Drawing for the job (mm, zero at the part's lowest x, y, z). A direction names the side the tool comes from. Give positions to 0.01 mm unless a question says otherwise; leave off trailing zeros. Write each loop counter-clockwise with the first axis right and the second up, starting at its lowest first coordinate (ties: lowest second). Pieces come first, ordered by that corner, then holes. Notation, with made-up numbers: (85, -24) - (127, -24) arc R25 ccw to (127, -3) - close; hole circle Ø2 at (77.5, 83.5). An arc over 180 degrees is marked (long way). Write item = value, one per line. Start each with the question number.
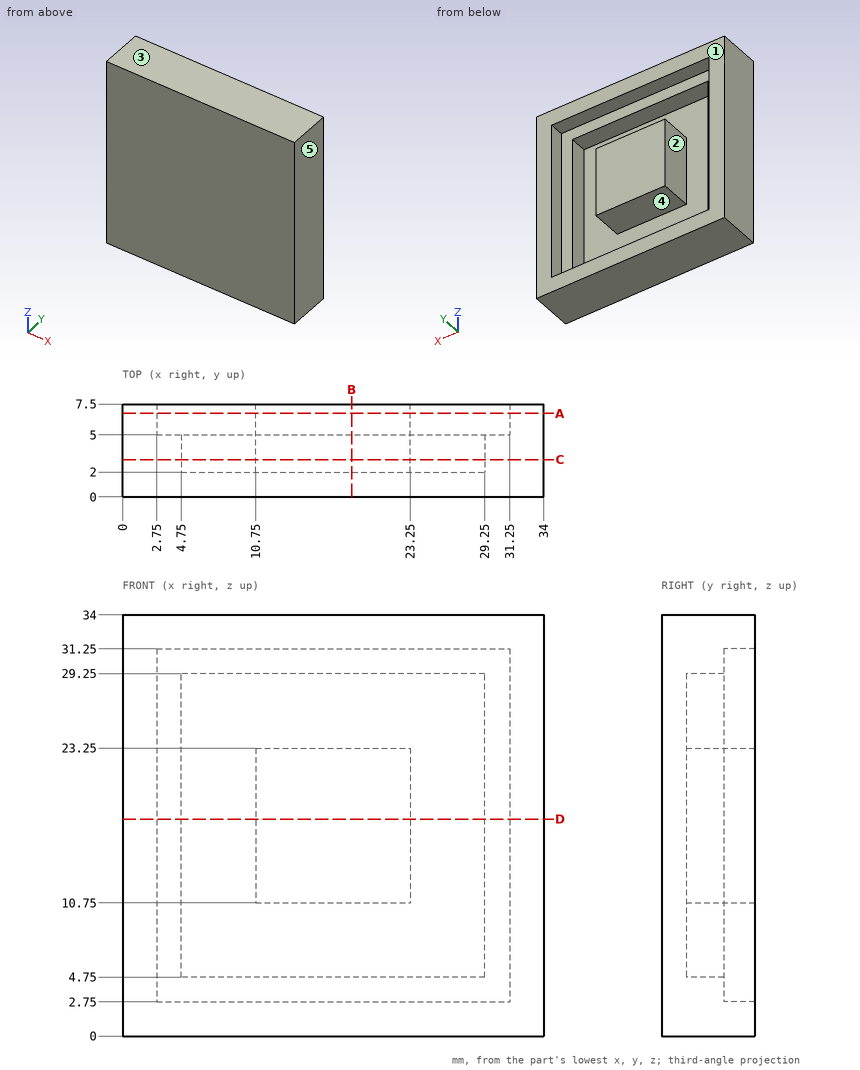
1. Cut at B-B (x = 18.5). Give the cut face in (y, z), then the cut area to 3 significant figures.
2. Tool access for the marked faces 1 and 2: list every direction of +Z, -Z, +X, -X, +Y, -Y with a clear straight run to the whole face (end or side of a thin tool).
3. Wall check: line 1 along X through (y, z) = (7.25, 14.5); line 2 along Z through (x, y) = (17, 4.5). Give the ranges that are in metal, low to high.
4. Cut at D-D (z = 17.5). Give the cut face in (x, y).
5. Pin check, flat tip, straight feed: pin 1 Ø3.5 at (x, y) = (17, 4) entering from -Z. Stop position of the tip, or through.
6. Cut at A-A (y = 6.75). Give the cut face in (x, z).
7. Cut at C-C (y = 3). Give the cut face in (x, z), then the cut area to 3 significant figures.
8. Mould opens along X. For the marked faces 3, 4 and 5 say: +X half, -X half, draft (parallel to the pull), parting line (faces both ways), or undercut.
Output:
q1.outline = (0, 0) - (7.5, 0) - (7.5, 2.75) - (5, 2.75) - (5, 4.75) - (2, 4.75) - (2, 10.75) - (7.5, 10.75) - (7.5, 23.25) - (2, 23.25) - (2, 29.25) - (5, 29.25) - (5, 31.25) - (7.5, 31.25) - (7.5, 34) - (0, 34) - close
q1.area = 179 mm2
q2.face_1 = +Z, -Z, +X, -X, +Y
q2.face_2 = +Y
q3.line_1 = 0 to 2.75, 10.75 to 23.25, 31.25 to 34
q3.line_2 = 0 to 4.75, 10.75 to 23.25, 29.25 to 34
q4.outline = (0, 0) - (34, 0) - (34, 7.5) - (31.25, 7.5) - (31.25, 5) - (29.25, 5) - (29.25, 2) - (23.25, 2) - (23.25, 7.5) - (10.75, 7.5) - (10.75, 2) - (4.75, 2) - (4.75, 5) - (2.75, 5) - (2.75, 7.5) - (0, 7.5) - close
q5.pin_1 = 0
q6.outline = (0, 0) - (34, 0) - (34, 34) - (0, 34) - close; (10.75, 10.75) - (23.25, 10.75) - (23.25, 23.25) - (10.75, 23.25) - close; hole (2.75, 2.75) - (31.25, 2.75) - (31.25, 31.25) - (2.75, 31.25) - close
q7.outline = (0, 0) - (34, 0) - (34, 34) - (0, 34) - close; (10.75, 10.75) - (23.25, 10.75) - (23.25, 23.25) - (10.75, 23.25) - close; hole (4.75, 4.75) - (29.25, 4.75) - (29.25, 29.25) - (4.75, 29.25) - close
q7.area = 712 mm2
q8.face_3 = draft
q8.face_4 = undercut
q8.face_5 = +X half
